from build123d import *

# Parameters (mm, degrees)
SKETCH1_R           = 1.25
BOSS_EXTRUDE1_DEPTH = 7
SKETCH2_R           = 4.5
BOSS_EXTRUDE2_DEPTH = 5
SKETCH3_R           = 4.5
BOSS_EXTRUDE3_DEPTH = 5
FILLET1_R           = 2
FILLET2_R           = 5


with BuildPart() as part:
    # Sketch1 → Boss-Extrude1 (new body)
    with BuildSketch(Plane(origin=(0, -692.732289503, 224.634763615), x_dir=(1, 0, 0), z_dir=(0, 0, -1))):
        Polygon((17.5, -2.476720525), (17.5, -34.476720525), (0, -42.476720525), (-17.5, -34.476720525), (-17.5, -2.476720525), align=None)
        with Locations(Location((-12.5, -27.476720525, 0), (0, 0, 270))):
            Circle(SKETCH1_R, mode=Mode.SUBTRACT)
        with Locations(Location((12.5, -27.476720525, 0), (0, 0, 270))):
            Circle(SKETCH1_R, mode=Mode.SUBTRACT)
        with Locations(Location((12.5, -7.476720525, 0), (0, 0, 270))):
            Circle(SKETCH1_R, mode=Mode.SUBTRACT)
        with Locations(Location((-12.5, -7.476720525, 0), (0, 0, 270))):
            Circle(SKETCH1_R, mode=Mode.SUBTRACT)
    extrude(amount=BOSS_EXTRUDE1_DEPTH)

    # Sketch2 → Boss-Extrude2 (add)
    with BuildSketch(Plane.XZ.offset(655.255568978)):
        with BuildLine():
            Line((6, 217.634763615), (-6, 217.634763615))
            Line((-6, 217.634763615), (-6, 211.634763615))
            ThreePointArc((-6, 211.634763615), (0, 205.634763615), (6, 211.634763615))
            Line((6, 211.634763615), (6, 217.634763615))
        make_face()
        with Locations(Location((0, 211.634763615, 0), (0, 0, 270))):
            Circle(SKETCH2_R, mode=Mode.SUBTRACT)
    extrude(amount=BOSS_EXTRUDE2_DEPTH)

    # Sketch3 → Boss-Extrude3 (add)
    with BuildSketch(Plane.XZ.offset(685.255568978)):
        with BuildLine():
            Line((6, 217.634763615), (-6, 217.634763615))
            Line((-6, 217.634763615), (-6, 211.634763615))
            ThreePointArc((-6, 211.634763615), (0, 205.634763615), (6, 211.634763615))
            Line((6, 211.634763615), (6, 217.634763615))
        make_face()
        with Locations(Location((0, 211.634763615, 0), (0, 0, 270))):
            Circle(SKETCH3_R, mode=Mode.SUBTRACT)
    extrude(amount=BOSS_EXTRUDE3_DEPTH)

    # Fillet1
    fillet1_edges = [part.edges().sort_by_distance(p)[0] for p in [
        (6, -657.755568978, 217.634763615),
        (-6, -657.755568978, 217.634763615),
        (6, -687.755568978, 217.634763615),
        (-6, -687.755568978, 217.634763615),
    ]]
    fillet(fillet1_edges, radius=FILLET1_R)

    # Fillet2
    fillet2_edges = [part.edges().sort_by_distance(p)[0] for p in [
        (17.5, -690.255568978, 221.134763615),
        (17.5, -658.255568978, 221.134763615),
        (0, -650.255568978, 221.134763615),
        (-17.5, -658.255568978, 221.134763615),
        (-17.5, -690.255568978, 221.134763615),
    ]]
    fillet(fillet2_edges, radius=FILLET2_R)


solid = part.part
Here's how the part is built. I have some questions about the finished solid (model axes, mm). A direction names the side the tool comes from. Round coordinates to 2 decimals unless told otherwise and drop trailing zeros. Write each loop counter-clockwise with the first axis right and the second up, starting at its lowest first coordinate (ties: lowest second). Pieces come first, ordered by that corner, then holes. Notation, with made-up numbers: (-16.75, -19) -> (14.25, -19) arc R15 ccw to (14.25, -2) -> close; hole circle Ø2 at (20.5, 52). An arc over 180 degrees is marked (long way). One line per item, written item: value.
1) I'm going to push flat-ended pins straight in: pin 1 Ø1.5 at (x, y) = (-12.5, -685.26) entering from +Z; pin 2 Ø3 at (x, z) = (-4, 218) entering from +Y; pin 3 Ø3 at (x, y) = (7, -681.5) entering from -Z; pin 4 Ø3 at (y, z) = (-657.5, 214.5) entering from +X. Where does each tip first touch, or does it pass through?
Filled sheet:
pin 1: passes through
pin 2: stops at y = -651.4
pin 3: stops at z = 217.63
pin 4: stops at x = 6.03
2) Suppose I cut it at B-B on z = 220.75. List the corners of the cut face in (x, y) for me.
Filled sheet:
outline: (-17.5, -685.26) arc R5 ccw to (-12.5, -690.26) -> (12.5, -690.26) arc R5 ccw to (17.5, -685.26) -> (17.5, -661.47) arc R5 ccw to (14.58, -656.92) -> (2.08, -651.21) arc R5 ccw to (-2.08, -651.21) -> (-14.58, -656.92) arc R5 ccw to (-17.5, -661.47) -> close; hole circle Ø2.5 at (-12.5, -685.26); hole circle Ø2.5 at (-12.5, -665.26); hole circle Ø2.5 at (12.5, -685.26); hole circle Ø2.5 at (12.5, -665.26)
3) Suppose I cut it at D-D on y = -687. List the corners of the cut face in (x, z) for me.
Filled sheet:
outline: (-17.19, 217.63) -> (-8, 217.63) arc R2 cw to (-6, 215.63) -> (-6, 211.63) arc R6 ccw to (6, 211.63) -> (6, 215.63) arc R2 cw to (8, 217.63) -> (17.19, 217.63) -> (17.19, 224.63) -> (-17.19, 224.63) -> close; hole circle Ø9 at (0, 211.63)
4) Suppose I cut it at C-C on z = 215. List the corners of the cut face in (x, y) for me.
Filled sheet:
outline: (-6, -690.26) -> (-2.99, -690.26) -> (-2.99, -685.26) -> (-6, -685.26) -> close; (-6, -660.26) -> (-2.99, -660.26) -> (-2.99, -655.26) -> (-6, -655.26) -> close; (2.99, -690.26) -> (6, -690.26) -> (6, -685.26) -> (2.99, -685.26) -> close; (2.99, -660.26) -> (6, -660.26) -> (6, -655.26) -> (2.99, -655.26) -> close
5) For faces 1 (the face through (2, -655.256, 216)), 2 (the face through (6, -688, 214)), 3 (the face through (-17.5, -673, 221)), which set-ups out of +Z, -Z, +X, -X, +Y, -Y let a thin tool reach every point of the face, with its end or its side?
Filled sheet:
face 1: -Z, +X, -X, +Y
face 2: -Z, +X, +Y, -Y
face 3: +Z, -Z, -X, +Y, -Y
6) If I drill on line 1 (Y direction, x = -2.5, z = 207.5); line 2 (X direction, y = -686, z = 221); line 3 (Z direction, x = 14, y = -664), over which ranges is the centre line in solid material (lowest first)? Write a range as [from, to].
Filled sheet:
line 1: y = [-690.26, -685.26], [-660.26, -655.26]
line 2: x = [-17.44, -13.5], [-11.5, 11.5], [13.5, 17.44]
line 3: z = [217.63, 224.63]
7) We'd pull the mould along Y, two halves only. Please class faces 4 (the face through (-15.996, -688.83, 221.086)), 5 (the face through (-1.724, -687.721, 207.478)), 6 (the face through (2, -660.256, 216)): released by +Y, released by -Y, zero draft, split by the parting line, or undercut.
Filled sheet:
face 4: released by -Y
face 5: zero draft
face 6: undercut
8) Suppose I cut it at A-A on x = 0. List the corners of the cut face in (y, z) for me.
Filled sheet:
outline: (-690.26, 205.63) -> (-685.26, 205.63) -> (-685.26, 207.13) -> (-690.26, 207.13) -> close; (-690.26, 216.13) -> (-685.26, 216.13) -> (-685.26, 217.63) -> (-660.26, 217.63) -> (-660.26, 216.13) -> (-655.26, 216.13) -> (-655.26, 217.63) -> (-650.75, 217.63) -> (-650.75, 224.63) -> (-690.26, 224.63) -> close; (-660.26, 205.63) -> (-655.26, 205.63) -> (-655.26, 207.13) -> (-660.26, 207.13) -> close
